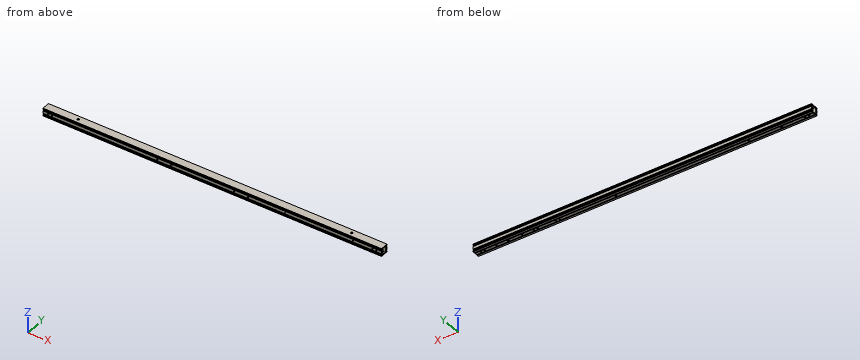
from build123d import *

# Parameters (mm, degrees)
SKETCH_1_W                = 23.5
SKETCH_1_H                = 12
EXTRUDE_1_DEPTH           = 650.5
HOLE_WIZARD_M6_1_D        = 5
HOLE_WIZARD_M6_1_DEPTH    = 19
HOLE_WIZARD_M6_1_TIP      = 1.502151548
HOLE_WIZARD_M6_2_D        = 5
HOLE_WIZARD_M6_2_DEPTH    = 19
HOLE_WIZARD_M6_2_TIP      = 1.502151548
HOLE_WIZARD_9_0_9_1_D     = 9
HOLE_WIZARD_7_0_7_1_D     = 7
HOLE_WIZARD_7_0_7_1_DEPTH = 15
HOLE_WIZARD_7_0_7_1_TIP   = 2.103012167
HOLE_WIZARD_M4_1_D        = 3.3
HOLE_WIZARD_M4_1_DEPTH    = 11.5
HOLE_WIZARD_M4_1_TIP      = 0.991420021


with BuildPart() as part:
    # 草图1 → 凸台-拉伸1 (new, symmetric)
    with BuildSketch(Plane(origin=(0, 0, 0), x_dir=(0, 0, -1), z_dir=(1, 0, 0))):
        Polygon((-15, 15), (-11.5, 15), (-11.5, 13.5), (-11, 13.5), (-11, 12), (-9.5, 12), (-9.5, 15), (-8, 15), (-8, 12.5), (-5, 12.5), (-5, 15), (5, 15), (5, 12.5), (8, 12.5), (8, 15), (9.5, 15), (9.5, 12), (11, 12), (11, 13.5), (11.5, 13.5), (11.5, 15), (15, 15), (15, 8), (12.5, 8), (12.5, 5), (15, 5), (15, -5), (12.5, -5), (12.5, -8), (15, -8), (15, -15), (11.5, -15), (11.5, -13.5), (11, -13.5), (11, -12), (9.5, -12), (9.5, -15), (8, -15), (8, -12.5), (5, -12.5), (5, -15), (-5, -15), (-5, -12.5), (-8, -12.5), (-8, -15), (-9.5, -15), (-9.5, -12), (-11, -12), (-11, -13.5), (-11.5, -13.5), (-11.5, -15), (-15, -15), align=None)
        with BuildLine():
            Line((12, -10.5), (12, -8.5))
            ThreePointArc((12, -8.5), (11.853553391, -8.146446609), (11.5, -8))
            Line((11.5, -8), (-11.5, -8))
            ThreePointArc((-11.5, -8), (-11.853553391, -8.146446609), (-12, -8.5))
            Line((-12, -8.5), (-12, -10.5))
            ThreePointArc((-12, -10.5), (-11.853553391, -10.853553391), (-11.5, -11))
            Line((-11.5, -11), (11.5, -11))
            ThreePointArc((11.5, -11), (11.853553391, -10.853553391), (12, -10.5))
        make_face(mode=Mode.SUBTRACT)
        with BuildLine():
            Line((-11.5, 11), (11.5, 11))
            ThreePointArc((11.5, 11), (11.853553391, 10.853553391), (12, 10.5))
            Line((12, 10.5), (12, 8.5))
            ThreePointArc((12, 8.5), (11.853553391, 8.146446609), (11.5, 8))
            Line((11.5, 8), (-11.5, 8))
            ThreePointArc((-11.5, 8), (-11.853553391, 8.146446609), (-12, 8.5))
            Line((-12, 8.5), (-12, 10.5))
            ThreePointArc((-12, 10.5), (-11.853553391, 10.853553391), (-11.5, 11))
        make_face(mode=Mode.SUBTRACT)
        Rectangle(SKETCH_1_W, SKETCH_1_H, mode=Mode.SUBTRACT)
    extrude(amount=EXTRUDE_1_DEPTH, both=True)

    # M6 螺纹孔1
    with Locations(Plane(origin=(0, 0, -15), x_dir=(-1, 0, 0), z_dir=(0, 0, -1))):
        with Locations((630.5, 0), (615.5, 0), (-327.5, 0), (-342.5, 0), (-412.5, 0), (-427.5, 0), (-615.5, 0), (-630.5, 0), (-570.5, 0), (-472.5, 0)):
            Hole(HOLE_WIZARD_M6_1_D / 2, depth=HOLE_WIZARD_M6_1_DEPTH)
            with Locations((0, 0, -(HOLE_WIZARD_M6_1_DEPTH + HOLE_WIZARD_M6_1_TIP / 2))):  # 118° drill point
                Cone(0, HOLE_WIZARD_M6_1_D / 2, HOLE_WIZARD_M6_1_TIP, mode=Mode.SUBTRACT)

    # M6 螺纹孔2
    with Locations(Plane(origin=(0, -15, 0), x_dir=(-1, 0, 0), z_dir=(0, -1, 0))):
        with Locations((-630.5, 0), (-615.5, 0), (615.5, 0), (630.5, 0), (-137.5, 0), (-83.5, 0), (157.5, 0), (211.5, 0)):
            Hole(HOLE_WIZARD_M6_2_D / 2, depth=HOLE_WIZARD_M6_2_DEPTH)
            with Locations((0, 0, -(HOLE_WIZARD_M6_2_DEPTH + HOLE_WIZARD_M6_2_TIP / 2))):  # 118° drill point
                Cone(0, HOLE_WIZARD_M6_2_D / 2, HOLE_WIZARD_M6_2_TIP, mode=Mode.SUBTRACT)

    # Ø9.0 (9) 直径孔1 (through all)
    with Locations(Plane.XY.offset(15)):
        with Locations((525.5, 0), (-525.5, 0)):
            Hole(HOLE_WIZARD_9_0_9_1_D / 2)

    # Ø7.0 (7) 直径孔1
    with Locations(Plane(origin=(0, 0, -15), x_dir=(-1, 0, 0), z_dir=(0, 0, -1))):
        with Locations((-111, 0), (399, 0)):
            Hole(HOLE_WIZARD_7_0_7_1_D / 2, depth=HOLE_WIZARD_7_0_7_1_DEPTH)
            with Locations((0, 0, -(HOLE_WIZARD_7_0_7_1_DEPTH + HOLE_WIZARD_7_0_7_1_TIP / 2))):  # 118° drill point
                Cone(0, HOLE_WIZARD_7_0_7_1_D / 2, HOLE_WIZARD_7_0_7_1_TIP, mode=Mode.SUBTRACT)

    # M4 螺纹孔1
    with Locations(Plane(origin=(0, -15, 0), x_dir=(-1, 0, 0), z_dir=(0, -1, 0))):
        with Locations((-540.5, 0), (-280.5, 0)):
            Hole(HOLE_WIZARD_M4_1_D / 2, depth=HOLE_WIZARD_M4_1_DEPTH)
            with Locations((0, 0, -(HOLE_WIZARD_M4_1_DEPTH + HOLE_WIZARD_M4_1_TIP / 2))):  # 118° drill point
                Cone(0, HOLE_WIZARD_M4_1_D / 2, HOLE_WIZARD_M4_1_TIP, mode=Mode.SUBTRACT)


solid = part.part
Could you check a few things on this model? Use its own coordinates, in mm. Give positions to 0.01 mm unless a question says otherwise; leave off trailing zeros. Answer as a JSON object with one key per item and string values.
Q1. Suppose I cut it at A-A on x = -238.5. Count the separate pieces of the cut face and the enclosed holes in it, then the cut area to 3 significant figures.
Taken from the geometry:
{"separate pieces": "1", "enclosed holes": "3", "area": "408 mm²"}
Q2. Please list where these lines run through material, in increasing order: L1, parallel to Y at x = 530, z = -6.75; L2, parallel to Y at x = 327.5, z = -13.7; L3, parallel to Y at x = -481, z = -13.25.
Taken from the geometry:
{"L1": "y = -12.5 to -11, -8 to -6, 6 to 8, 11 to 12.5", "L2": "y = -15 to -8, -5 to -2.5, 2.5 to 5, 8 to 15", "L3": "y = -15 to -8, -5 to 5, 8 to 15"}
Q3. Will these pins go through, and if not, where does the flat tip stop? pin 1 Ø4.5 at (x, y) = (327.5, 0) entering from -Z; pin 2 Ø1 at (x, y) = (-405.5, -6) entering from -Z; pin 3 Ø12 at (x, z) = (-422.5, 7.5) entering from +Y; pin 4 Ø1.6 at (x, z) = (-162.5, 10.5) entering from -Y.
Taken from the geometry:
{"pin 1": "stops at z = 11.75", "pin 2": "stops at z = -12.5", "pin 3": "stops at y = 15", "pin 4": "stops at y = -13.5"}
